The listing builds one solid part. Answer for the finished solid, in the listing's coordinates (mm). A direction names the side the tool comes from. Give positions to 0.01 mm unless a question says otherwise; leave off trailing zeros. Write each loop counter-clockwise with the first axis right and the second up, starting at its lowest first coordinate (ties: lowest second). Pieces come first, ordered by that corner, then holes. Notation, with made-up numbers: M 24,73 L 71,73 A25 ccw 71,101 Z; hole C -27.5,-29 d9. An arc over 180 degrees is marked long. Return JSON: item names as keys, results as strings.
from build123d import *

# Parameters (mm, degrees)
SKETCH3_R           = 8
BOSS_EXTRUDE1_DEPTH = 6
SKETCH4_R           = 4
CUT_EXTRUDE1_DEPTH  = 7
CIRPATTERN2_COUNT   = 10
RIB1_REACH          = 88.938
SKETCH2_WALL_W      = 205.405027826
SKETCH2_WALL_H      = 3
CIRPATTERN1_COUNT   = 10
RIB2_REACH          = 52
SKETCH5_WALLS_W     = 128
SKETCH5_WALLS_H     = 3
CIRPATTERN3_COUNT   = 10


with BuildPart() as part:
    # Sketch1 → Revolve1 (revolve)
    with BuildSketch(Plane.XY, mode=Mode.PRIVATE) as revolve1_sk:
        Polygon((34, 0), (34, 50), (40, 50), (40, 28), (66, 28), (66, 35), (72, 35), (72, 6), (83, 6), (83, 0), (66, 0), (66, 22), (40, 22), (40, 0), align=None)
    revolve(revolve1_sk.sketch.rotate(Axis((0, 0, 0), (0, 1, 0)), 90), axis=Axis((0, 0, 0), (0, 1, 0)))  # turned: the seam where the file's is

    # Sketch3 → Boss-Extrude1 (add)
    with BuildSketch(Plane(origin=(0, 6, 0), x_dir=(1, 0, 0), z_dir=(0, 1, 0))):
        with Locations((-83, 0)):
            Circle(SKETCH3_R)
    boss_extrude1 = extrude(amount=-BOSS_EXTRUDE1_DEPTH)

    # Sketch4 → Cut-Extrude1 (cut, through all)
    with BuildSketch(Plane(origin=(0, 6, 0), x_dir=(1, 0, 0), z_dir=(0, 1, 0))):
        with Locations(Location((-83, 0, 0), (0, 0, 270))):  # turned: the seam where the file's is
            Circle(SKETCH4_R)
    cut_extrude1 = extrude(amount=-CUT_EXTRUDE1_DEPTH, mode=Mode.SUBTRACT)

    # CirPattern2: Boss-Extrude1, Cut-Extrude1 ×10 about axis
    cirpattern2_axis = Axis((0, 0, 0), (0, 1, 0))
    add([boss_extrude1.rotate(cirpattern2_axis, i * 360 / CIRPATTERN2_COUNT) for i in range(1, CIRPATTERN2_COUNT)])
    add([cut_extrude1.rotate(cirpattern2_axis, i * 360 / CIRPATTERN2_COUNT) for i in range(1, CIRPATTERN2_COUNT)], mode=Mode.SUBTRACT)

    # Sketch2 wall → Rib1 (add, up to next)
    with BuildSketch(Plane(origin=(-53, 38, 0), x_dir=(-0.8804711, -0.474099823, 0), z_dir=(0.474099823, -0.8804711, 0)), mode=Mode.PRIVATE) as rib1_sk1:
        Rectangle(SKETCH2_WALL_W, SKETCH2_WALL_H)
    rib1_tool1 = extrude(rib1_sk1.sketch, amount=RIB1_REACH, mode=Mode.PRIVATE) - part.part
    rib1 = rib1_tool1.solids().sort_by_distance((-53, 38, 0))[0]
    add(rib1)

    # CirPattern1: Rib1 ×10 about axis
    cirpattern1_axis = Axis((0, 0, 0), (0, 1, 0))
    for i in range(1, CIRPATTERN1_COUNT):
        add(rib1.rotate(cirpattern1_axis, i * 360 / CIRPATTERN1_COUNT))

    # Sketch5 walls → Rib2 (add, up to next)
    with BuildSketch(Plane.XZ, mode=Mode.PRIVATE) as rib2_sk1:
        with Locations((-53, 0)):
            Rectangle(SKETCH5_WALLS_W, SKETCH5_WALLS_H)
    rib2_tool1 = extrude(rib2_sk1.sketch, amount=-RIB2_REACH, mode=Mode.PRIVATE) - part.part
    rib2 = rib2_tool1.solids().sort_by_distance((-53, 0, 0))[0]
    add(rib2)

    # CirPattern3: Rib2 ×10 about axis
    cirpattern3_axis = Axis((0, 0, 0), (0, -1, 0))
    for i in range(1, CIRPATTERN3_COUNT):
        add(rib2.rotate(cirpattern3_axis, i * 360 / CIRPATTERN3_COUNT))


solid = part.part
Item 1: A cutting plane is placed at C-C, the plane x = 60. Write down the section's boundary in (y, z), plus the area to 3 significant figures.
Geometry results:
{"outline": "M 0,-57.35 L 6,-57.35 L 6,-39.8 L 35,-39.8 L 35,-27.5 L 28,-27.5 L 28,-1.5 L 34.23,-1.5 L 34.23,1.5 L 28,1.5 L 28,27.5 L 35,27.5 L 35,39.8 L 6,39.8 L 6,57.35 L 0,57.35 L 0,27.5 L 22,27.5 L 22,1.5 L 0,1.5 L 0,-1.5 L 22,-1.5 L 22,-27.5 L 0,-27.5 Z", "area": "1,490 mm2"}
Item 2: Which of the six approach directions +Z, -Z, +X, -X, +Y, -Y give full straight-line access (tool end or side, diameter ignored) to faces 4 (the flat face through (-41.9, 32.74, 28.59)), 5 (the cylindrical face through (71.1, 3, 49.4)), 6 (the cylindrical face through (-23.39, 10.85, -32.45))?
Geometry results:
{"face 4": "+Y", "face 5": "+Y, -Y", "face 6": "-Y"}
Item 3: A cutting plane is placed at B-B, the plane z = -14. Write down the section's boundary in (x, y).
Geometry results:
{"outline": "M -81.81,0 L -64.5,0 L -64.5,22 L -37.47,22 L -37.47,0 L -30.98,0 L -30.98,50 L -37.47,50 L -37.47,28 L -64.5,28 L -64.5,35 L -70.63,35 L -70.63,6 L -81.81,6 Z; M 30.98,0 L 37.47,0 L 37.47,22 L 64.5,22 L 64.5,0 L 81.81,0 L 81.81,6 L 70.63,6 L 70.63,35 L 64.5,35 L 64.5,28 L 37.47,28 L 37.47,50 L 30.98,50 Z"}
Item 4: Find the intervals of material crossed by line 1 (X direction, y = 15, z = 8); line 2 (X direction, y = 26, z = 1.5); line 3 (Z direction, x = -42, y = 14.5), in increasing order.
Geometry results:
{"line 1": "x = -71.55 to -65.51, -39.19 to -33.05, 33.05 to 39.19, 65.51 to 71.55", "line 2": "x = -71.98 to -33.97, 33.97 to 71.98", "line 3": "z = -58.48 to -50.91, -32.37 to -28.66, -1.5 to 1.5, 28.66 to 32.37, 50.91 to 58.48"}
Item 5: Determine the mould class of faces 1 (the cylindrical face through (-28.29, 3.04, 86.49)), 2 (the flat face through (17.094, 32.739, 47.757)), 3 (the cylindrical face through (78.86, 2.96, 25.89)) for opening direction X: +X half, -X half, draft (parallel to the pull), parting line (faces both ways), or undercut.
Geometry results:
{"face 1": "undercut", "face 2": "undercut", "face 3": "+X half"}
Item 6: A cutting plane is placed at A-A, the plane x = 0. Write down the section's boundary in (y, z), plus the area to 3 significant figures.
Geometry results:
{"outline": "M 0,-83 L 6,-83 L 6,-72 L 35,-72 L 35,-66 L 28,-66 L 28,-40 L 50,-40 L 50,-34 L 0,-34 L 0,-40 L 22,-40 L 22,-66 L 0,-66 Z; M 0,34 L 50,34 L 50,40 L 28,40 L 28,66 L 35,66 L 35,72 L 6,72 L 6,83 L 0,83 L 0,66 L 22,66 L 22,40 L 0,40 Z", "area": "1,460 mm2"}
Item 7: Given pin 1 Ø2 at (x, z) = (-47.5, 24.5) entering from -Y; pin 2 Ø14 at (x, z) = (9, 57) entering from +Y; pin 3 Ø10.5 at (x, z) = (-67.15, -48.79) entering from +Y, each flat-ended and moving along its own axis, determine where each tip first touches the part or whether it passes through.
Geometry results:
{"pin 1": "stops at y = 22", "pin 2": "stops at y = 28", "pin 3": "stops at y = 6"}
